```python
from build123d import *

# Parameters (mm, degrees)
BOSS_EXTRUDE1_DEPTH  = 4.7625
FILLET1_R            = 1.27
M6_CLEARANCE_HOLE1_D = 6.6


with BuildPart() as part:
    # Sketch1 → Boss-Extrude1 (new body)
    with BuildSketch(Plane(origin=(0, 0, 0), x_dir=(1, 0, 0), z_dir=(0, 1, 0))):
        with BuildLine():
            Line((-29.505035319724954, 4.784524777155699), (-7.166713759633276, -10.484665654539652))
            ThreePointArc((-7.166713759633276, -10.484665654539652), (-11.24843137291464, 5.895997934941107), (4.544931572497542, 11.8589037014943))
            Line((4.544931572497542, 11.8589037014943), (-20.721301320626843, 21.542201794181164))
            ThreePointArc((-20.721301320626843, 21.542201794181164), (-32.56632352968598, 17.07002246926627), (-29.505035319724954, 4.784524777155699))
        make_face()
    extrude(amount=BOSS_EXTRUDE1_DEPTH)

    # Fillet1
    fillet1_edges = [part.edges().sort_by_distance(p)[0] for p in [
        (4.544931572497541, 2.38125, -11.858903701494302),
        (-7.166713759633276, 2.38125, 10.484665654539652),
    ]]
    fillet(fillet1_edges, radius=FILLET1_R)

    # M6 Clearance Hole1 (through all)
    with Locations(Plane(origin=(0, 4.7625, 0), x_dir=(1, 0, 0), z_dir=(0, 1, 0))):
        with Locations((-24.13, 12.648024018)):
            Hole(M6_CLEARANCE_HOLE1_D / 2)


solid = part.part
```
Input: part model. Units: mm. Frame: model coordinates. Coordinates: 2 decimals unless noted, no trailing zeros. Order: outer loops, then holes, each group sorted by start corner. A loop starts at its lowest first (then second) coordinate and runs counter-clockwise, first axis right, second up. Notation, with made-up numbers: (21, 45.5) - (41, 45.5) arc R17 ccw to (41, 53.5) - close; hole circle Ø7 at (52.5, 56). An arc over 180 degrees is marked (long way). Put each result on its own line as item: value.
1. Draft query along Z for faces 1 (the face through (-2.144, 2.415, -13.449)), 2 (the face through (-11.71, 2.35, -18.09)), 3 (the face through (-27.178, 2.348, -11.384)). Return one class per face: pulls with the +Z half, pulls with the -Z half, needs draft (parallel to the pull), parting line crosses it, or undercut.
Report:
face 1: parting line crosses it
face 2: pulls with the -Z half
face 3: undercut
2. Cut plane C-C on z = -18.25. Return the cut outline in (x, y), then the cut area to 3 significant figures.
Report:
outline: (-31.83, 0) - (-12.13, 0) - (-12.13, 4.76) - (-31.83, 4.76) - close
area: 93.8 mm2
3. Cut plane B-B on y = 0.5. Return the cut outline in (x, z) (3 decimals).
Report:
outline: (-29.505, -4.785) arc R9.525 ccw to (-20.721, -21.542) - (-2.955, -14.733) arc R1.27 ccw to (-3.1, -12.316) arc R12.7 cw to (-11.892, 4.458) arc R1.27 ccw to (-13.798, 5.952) - close; hole circle Ø6.6 at (-24.13, -12.648)
4. Cut plane A-A on x = -24.13. Return the cut outline in (y, z), then the cut area to 3 significant figures.
Report:
outline: (0, -22.17) - (4.76, -22.17) - (4.76, -15.95) - (0, -15.95) - close; (0, -9.35) - (4.76, -9.35) - (4.76, -1.11) - (0, -1.11) - close
area: 68.9 mm2
5. Line query: line 1 along Z through (x, y) = (-27, 3.6); line 2 along X through (y, z) = (4.25, -12.75); line 3 along X through (y, z) = (2.9, -14.25). Output: solid intervals per line, ascending.
Report:
line 1: z = -21.73 to -14.28, -11.02 to -3.07
line 2: x = -33.65 to -27.43, -20.83 to -2.42
line 3: x = -33.52 to -27.02, -21.24 to -2.35
6. Contact query for flat-ended pins moving along their axis: pin 1 Ø2 at (y, z) = (2.5, -16.5) entering from -X; pin 2 Ø6 at (x, z) = (-24.13, -12.65) entering from -Y. Output: stop coordinate, or through.
Report:
pin 1: stops at x = -33.22
pin 2: passes through
7. Cut plane D-D on x = -18.5. Return the cut outline in (y, z), then the cut area to 3 significant figures.
Report:
outline: (0, -20.69) - (4.76, -20.69) - (4.76, 2.74) - (0, 2.74) - close
area: 112 mm2
